```python
from build123d import *

# Parameters (mm, degrees)
F0_R      = 1.7145
F0_W      = 48.26
F0_H      = 10.4902
F1_DEPTH  = 3.175
F2_W      = 55.88
F2_H      = 36.83
F3_DEPTH  = 11.1252
F5_DEPTH  = 14.3012
F6_W      = 55.88
F6_H      = 3.175
F7_DEPTH  = 9.525
F8_R      = 1.016
F9_DEPTH  = 105.1062
F10_W     = 30.48
F10_H     = 7.9502
F11_DEPTH = 52.07
F12_R     = 3.175
F13_R     = 1.7145
F14_DEPTH = 25.4
F16_DEPTH = 10.16


with BuildPart() as f1:
    # F0 (on Top) → F1 (new body)
    with BuildSketch(Plane.XY):
        Polygon((-27.94, 0), (27.94, 0), (27.94, 72.39), (27.94, 95.5802), (-27.94, 95.5802), (-27.94, 72.39), align=None)
        with Locations((-9.8679, 58.0898)):
            Circle(F0_R, mode=Mode.SUBTRACT)
        with Locations((0, 80.8101)):
            Rectangle(F0_W, F0_H, mode=Mode.SUBTRACT)
        with Locations((-9.8679, 90.8177)):
            Circle(F0_R, mode=Mode.SUBTRACT)
        with Locations((9.8679, 58.0898)):
            Circle(F0_R, mode=Mode.SUBTRACT)
        with Locations((9.8679, 90.8177)):
            Circle(F0_R, mode=Mode.SUBTRACT)
    extrude(amount=F1_DEPTH)

    # F2 (on face) → F3 (join)
    with BuildSketch(Plane(origin=(0, 0, 0), x_dir=(1, 0, 0), z_dir=(0, 0, -1))):
        with Locations((0, -18.415)):
            Rectangle(F2_W, F2_H)
    extrude(amount=F3_DEPTH)

    # F4 (on face) → F5 (cut, through all)
    with BuildSketch(Plane(origin=(0, 0, -11.1252), x_dir=(1, 0, 0), z_dir=(0, 0, -1))):
        with BuildLine():
            Line((-27.94, -6.35), (-27.94, -21.59))
            Line((-27.94, -21.59), (-18.415, -21.59))
            ThreePointArc((-18.415, -21.59), (-10.795, -13.97), (-18.415, -6.35))
            Line((-18.415, -6.35), (-27.94, -6.35))
        make_face()
    extrude(amount=-F5_DEPTH, mode=Mode.SUBTRACT)

    # F6 (on face) → F7 (join)
    with BuildSketch(Plane.XZ):
        with Locations((0, 1.5875)):
            Rectangle(F6_W, F6_H)
    extrude(amount=F7_DEPTH)

    # F8 (on face) → F9 (cut, through all)
    with BuildSketch(Plane(origin=(0, 95.5802, 0), x_dir=(-1, 0, 0), z_dir=(0, 1, 0))):
        with Locations((0, 3.175)):
            Circle(F8_R)
    extrude(amount=-F9_DEPTH, mode=Mode.SUBTRACT)

    # F10 (on face) → F11 (cut)
    with BuildSketch(Plane(origin=(-27.94, 0, 0), x_dir=(0, -1, 0), z_dir=(-1, 0, 0))):
        with Locations((-18.415, -3.9751)):
            Rectangle(F10_W, F10_H)
    extrude(amount=-F11_DEPTH, mode=Mode.SUBTRACT)

    # F12
    f12_edges = [f1.edges().sort_by_distance(p)[0] for p in [
        (24.13, 75.565, 1.5875),
        (-24.13, 75.565, 1.5875),
        (-24.13, 86.0552, 1.5875),
        (24.13, 86.0552, 1.5875),
    ]]
    fillet(f12_edges, radius=F12_R)

    # F13 (on face) → F14 (cut)
    with BuildSketch(Plane(origin=(0, 0, 0), x_dir=(1, 0, 0), z_dir=(0, 0, -1))):
        with Locations((-9.8679, 4.7625)):
            Circle(F13_R)
        with Locations((9.8679, 4.7625)):
            Circle(F13_R)
    extrude(amount=-F14_DEPTH, mode=Mode.SUBTRACT)

    # F15 (on face) → F16 (cut)
    with BuildSketch(Plane(origin=(0, 0, -11.1252), x_dir=(1, 0, 0), z_dir=(0, 0, -1))):
        with BuildLine():
            Line((-6.35, -36.83), (6.35, -36.83))
            ThreePointArc((6.35, -36.83), (0, -30.48), (-6.35, -36.83))
        make_face()
    extrude(amount=-F16_DEPTH, mode=Mode.SUBTRACT)


solid = f1.part
```
Build history of the part. All positions in model axes, mm. A direction names the side the tool comes from. Give positions to 0.01 mm unless a question says otherwise; leave off trailing zeros. Order: outer loops, then holes, each group sorted by start corner. A loop starts at its lowest first (then second) coordinate and runs counter-clockwise, first axis right, second up. Notation, with made-up numbers: M 71,9 L 120,9 A28 ccw 120,44 Z; hole C -3.5,64 d4. An arc over 180 degrees is marked long. Write item = value, one per line. Start each with the question number.
(1) Which spindle directions (+Z, -Z, +X, -X, +Y, -Y) get a long thin tool onto all of the face, cutting with end or side? Do faces 1 (the flat face through (-23, 6.35, 2)), 2 (the cylindrical face through (0.02, 33.62, 2.16)), 3 (the flat face through (24.13, 81, 2)), 4 (the flat face through (0, 0, -5)), 5 (the flat face through (24.13, 19, -4)). Say none if no direction does.
(2) Slice it at D-D on z = -2.5. Write the cut outline in (x, y) (3 decimals), plus the area to 3 significant figures.
(3) Slice it at C-C on y = 26. Write the cut outline in (x, z) (3 decimals).
(4) Probe L1, parallel to Y at x = -4.5, z = 1 (3 decimals); L2, parallel to Y at x = -10, z = -6.5 (3 decimals); L3, parallel to Z at x = -20, y = 4 (3 decimals). List the from-to ranges inside material, lowest first. Write a range as [from, to].
(5) Two-plate mould, pull along Z, no slides. Class faces 6 (the flat face through (14, 44, 3.175)), 7 (the flat face through (-27.94, 53.3, 0.3)), 8 (the flat face through (4, 19, -7.95)): released by +Z, released by -Z, zero draft, split by the parting line, or undercut.
(6) Pin check, flat tips, straight feed: pin 1 Ø2.5 at (x, y) = (2.5, 36) entering from -Z; pin 2 Ø3.5 at (x, z) = (-22.5, -10) entering from +Y; pin 3 Ø4 at (x, z) = (-22, -7) entering from -Y; pin 4 Ø2.5 at (x, y) = (9.87, 58.09) entering from -Z. Stop position of each tip, or through.
(7) Slice it at A-A on x = 0. Write the cut outline in (y, z) (3 decimals), plus the area to 3 significant figures.
(8) Slice it at B-B on x = -19.5. Write the cut outline in (y, z) (3 decimals).
Responses:
q1.face_1 = +Z, -Z, -X
q1.face_2 = +Z, +Y, -Y
q1.face_3 = +Z, -Z
q1.face_4 = -Z, +X, -X, -Y
q1.face_5 = -X
q2.outline = M -27.94,0 L 27.94,0 L 27.94,36.83 L 6.35,36.83 A6.35 cw 5.499,33.655 L 24.13,33.655 L 24.13,3.175 L -27.94,3.175 Z; M -27.94,33.655 L -5.499,33.655 A6.35 cw -6.35,36.83 L -27.94,36.83 Z
q2.area = 432 mm2
q3.outline = M -27.94,-11.125 L 27.94,-11.125 L 27.94,3.175 L 1.016,3.175 A1.016 cw -1.016,3.175 L -27.94,3.175 L -27.94,0 L 24.13,0 L 24.13,-7.95 L -27.94,-7.95 Z
q4.L1 = [-9.525, 75.565], [86.055, 95.58]
q4.L2 = [0, 3.175], [33.655, 36.83]
q4.L3 = [-11.125, -7.95], [0, 3.175]
q5.face_6 = released by +Z
q5.face_7 = zero draft
q5.face_8 = undercut
q6.pin_1 = -0.97
q6.pin_2 = 36.83
q6.pin_3 = 0
q6.pin_4 = through
q7.outline = M -9.525,0 L 0,0 L 0,-11.125 L 30.48,-11.125 L 30.48,-7.95 L 3.175,-7.95 L 3.175,0 L 33.655,0 L 33.655,-0.965 L 36.83,-0.965 L 36.83,0 L 75.565,0 L 75.565,2.159 L -9.525,2.159 Z; M 86.055,0 L 95.58,0 L 95.58,2.159 L 86.055,2.159 Z
q7.area = 329 mm2
q8.outline = M -9.525,0 L 0,0 L 0,-11.125 L 6.35,-11.125 L 6.35,-7.95 L 3.175,-7.95 L 3.175,0 L 6.35,0 L 6.35,3.175 L -9.525,3.175 Z; M 21.59,-11.125 L 36.83,-11.125 L 36.83,0 L 75.565,0 L 75.565,3.175 L 21.59,3.175 L 21.59,0 L 33.655,0 L 33.655,-7.95 L 21.59,-7.95 Z; M 86.055,0 L 95.58,0 L 95.58,3.175 L 86.055,3.175 Z
